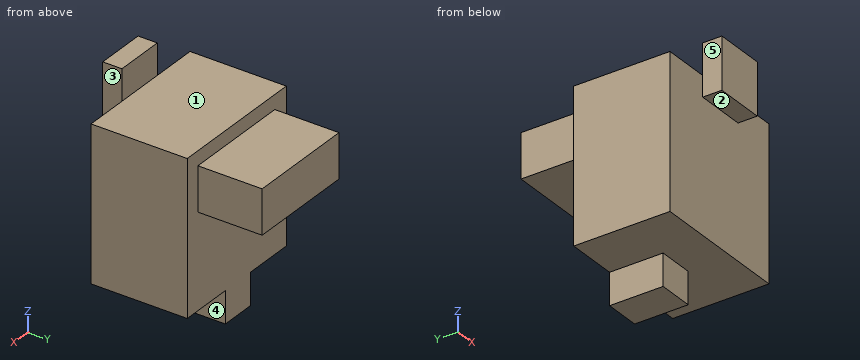
```python
from build123d import *

# Parameters (mm, degrees)
SKETCH1_W           = 39.91
SKETCH1_H           = 43.12
BOSS_EXTRUDE1_DEPTH = 27.2
SKETCH2_W           = 10.1
SKETCH2_H           = 15.13
BOSS_EXTRUDE2_DEPTH = 9
SKETCH5_W           = 14.25
SKETCH5_H           = 14.62
BOSS_EXTRUDE3_DEPTH = 5.43
SKETCH6_W           = 30.97
SKETCH6_H           = 12.5
BOSS_EXTRUDE4_DEPTH = 18.15


with BuildPart() as part:
    # Sketch1 → Boss-Extrude1 (new body)
    with BuildSketch(Plane(origin=(0, 0, 0), x_dir=(1, 0, 0), z_dir=(0, 1, 0))):
        Rectangle(SKETCH1_W, SKETCH1_H)
    extrude(amount=BOSS_EXTRUDE1_DEPTH)

    # Sketch2 → Boss-Extrude2 (add)
    with BuildSketch(Plane(origin=(0, 0, -21.56), x_dir=(-1, 0, 0), z_dir=(0, 0, -1))):
        with Locations((0.445, 19.635)):
            Rectangle(SKETCH2_W, SKETCH2_H)
    extrude(amount=BOSS_EXTRUDE2_DEPTH)

    # Sketch5 → Boss-Extrude3 (add)
    with BuildSketch(Plane.XZ):
        with Locations((0.36, 23.01)):
            Rectangle(SKETCH5_W, SKETCH5_H)
    extrude(amount=BOSS_EXTRUDE3_DEPTH)

    # Sketch6 → Boss-Extrude4 (add)
    with BuildSketch(Plane(origin=(0, 27.2, 0), x_dir=(1, 0, 0), z_dir=(0, 1, 0))):
        with Locations((0.17, -11.254639855)):
            Rectangle(SKETCH6_W, SKETCH6_H)
    extrude(amount=BOSS_EXTRUDE4_DEPTH)


solid = part.part
```
Input: part model. Units: mm. Frame: model coordinates. Face numbers are marked on the shaded views. A direction names the side the tool comes from. Coordinates: 2 decimals unless noted, no trailing zeros. Loops run counter-clockwise (first coordinate to the right, second up) from the corner with the lowest first, then second, coordinate; pieces in that order, holes last. Notation, with made-up numbers: (6, 83.25) -> (46, 83.25) arc R27 cw to (46, 107.25) -> close; hole circle Ø8 at (7, -17.5). An arc over 180 degrees is marked (long way). Use a Markdown table: item, result.
1) Cut plane C-C (z = 19). Return the cut outline in (x, y) (3 decimals), then the cut area to 3 significant figures.
Results found:
| item | result |
|---|---|
| outline | (-19.955, 0) -> (-6.765, 0) -> (-6.765, -5.43) -> (7.485, -5.43) -> (7.485, 0) -> (19.955, 0) -> (19.955, 27.2) -> (-19.955, 27.2) -> close |
| area | 1,160 mm2 |
2) Cut plane B-B (y = 25.5). Return the cut outline in (x, z) (3 decimals).
Results found:
| item | result |
|---|---|
| outline | (-19.955, -21.56) -> (-5.495, -21.56) -> (-5.495, -30.56) -> (4.605, -30.56) -> (4.605, -21.56) -> (19.955, -21.56) -> (19.955, 21.56) -> (-19.955, 21.56) -> close |
3) Cut plane A-A (x = 2.5). Return the cut outline in (y, z).
Results found:
| item | result |
|---|---|
| outline | (-5.43, 15.7) -> (0, 15.7) -> (0, -21.56) -> (12.07, -21.56) -> (12.07, -30.56) -> (27.2, -30.56) -> (27.2, 5) -> (45.35, 5) -> (45.35, 17.5) -> (27.2, 17.5) -> (27.2, 21.56) -> (0, 21.56) -> (0, 30.32) -> (-5.43, 30.32) -> close |
4) Material intervals for line 1 along Y through (x, z) = (-17.5, 0); line 2 along Z through (x, y) = (14, 25); line 3 along Z through (x, y) = (6.5, 37), sorted ascending. Write a range as from..to.
Results found:
| item | result |
|---|---|
| line 1 | y = 0..27.2 |
| line 2 | z = -21.56..21.56 |
| line 3 | z = 5..17.5 |
5) Cut plane D-D (z = -23). Return the cut outline in (x, y) (3 decimals), then the cut area to 3 significant figures.
Results found:
| item | result |
|---|---|
| outline | (-5.495, 12.07) -> (4.605, 12.07) -> (4.605, 27.2) -> (-5.495, 27.2) -> close |
| area | 153 mm2 |
6) Access query for the marked faces 1, 2, 3, 4 and 5. Directions: +Z, -Z, +X, -X, +Y, -Y. A direction counts if a zero-diameter tool reaches every point of the face in a straight line with its end or side. Return the directions, or none.
Results found:
| item | result |
|---|---|
| face 1 | +Z, +X, -X, +Y |
| face 2 | -Z, +X, -X, -Y |
| face 3 | +Z, -Z, +X, -Y |
| face 4 | -Z, +X, +Y, -Y |
| face 5 | +Z, -Z, -X, -Y |
7) Contact query for flat-ended pins moving along their axis: pin 1 (2.5 mm diameter, centred on y = 23.5, z = -28, fed in from +X) (3 decimals); pin 2 (8 mm diameter, centred on x = 11.5, y = 15.5, fed in from -Z); pin 3 (9.5 mm diameter, centred on x = 2.5, z = 27.5, fed in from +Y); pin 4 (8 mm diameter, centred on y = 32, z = -5, fed in from -X). Output: stop coordinate, or through.
Results found:
| item | result |
|---|---|
| pin 1 | stops at x = 4.605 |
| pin 2 | stops at z = -21.56 |
| pin 3 | stops at y = 0 |
| pin 4 | passes through |
